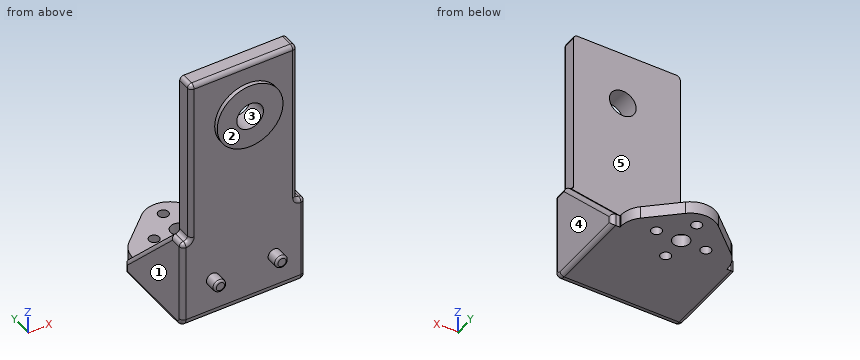
from build123d import *

# Parameters (mm, degrees)
SKETCH1_R           = 2
SKETCH1_R_2         = 1.25
BOSS_EXTRUDE1_DEPTH = 3
SKETCH2_W           = 26
SKETCH2_H           = 4
BOSS_EXTRUDE2_DEPTH = 60
SKETCH3_R           = 3.25
CUT_EXTRUDE1_DEPTH  = 72.226350639
SKETCH4_R           = 8
SKETCH4_R_2         = 3.25
BOSS_EXTRUDE3_DEPTH = 1
SKETCH5_R           = 1.5
BOSS_EXTRUDE4_DEPTH = 3
BOSS_EXTRUDE5_DEPTH = 2
FILLET1_R           = 2
FILLET2_R           = 1
FILLET3_R           = 0.5


# Some blends are built 0.0001 mm under size
with BuildPart() as part:
    # Sketch1 → Boss-Extrude1 (new body)
    with BuildSketch(Plane.XY):
        with BuildLine():
            Line((-13, -2.68256679), (-13, -25))
            Line((-13, -25), (13, -25))
            Line((13, -25), (13, -2.68256679))
            ThreePointArc((13, -2.68256679), (12.477468733, -0.233620837), (11.000887907, 1.788774838))
            Line((11.000887907, 1.788774838), (4.000887907, 8.052267471))
            ThreePointArc((4.000887907, 8.052267471), (0, 9.580925842), (-4.000887907, 8.052267471))
            Line((-4.000887907, 8.052267471), (-11.000887907, 1.788774838))
            ThreePointArc((-11.000887907, 1.788774838), (-12.477468733, -0.233620837), (-13, -2.68256679))
        make_face()
        Circle(SKETCH1_R, mode=Mode.SUBTRACT)
        with Locations((-6, 0)):
            Circle(SKETCH1_R_2, mode=Mode.SUBTRACT)
        with Locations((0, 6)):
            Circle(SKETCH1_R_2, mode=Mode.SUBTRACT)
        with Locations((6, 0)):
            Circle(SKETCH1_R_2, mode=Mode.SUBTRACT)
        with Locations((0, -6)):
            Circle(SKETCH1_R_2, mode=Mode.SUBTRACT)
    extrude(amount=BOSS_EXTRUDE1_DEPTH)

    # Sketch2 → Boss-Extrude2 (add)
    with BuildSketch(Plane.XY.offset(3)):
        with Locations((0, -23)):
            Rectangle(SKETCH2_W, SKETCH2_H)
    extrude(amount=BOSS_EXTRUDE2_DEPTH)

    # Sketch3 → Cut-Extrude1 (cut, through all)
    with BuildSketch(Plane(origin=(0, -21, 0), x_dir=(1, 0, 0), z_dir=(0, 1, 0))):
        with Locations(Location((1, -50, 0), (0, 0, 270))):
            Circle(SKETCH3_R)
    extrude(amount=-CUT_EXTRUDE1_DEPTH, mode=Mode.SUBTRACT)

    # Sketch4 → Boss-Extrude3 (add)
    with BuildSketch(Plane.XZ.offset(25)):
        with Locations(Location((1, 50, 0), (0, 0, 180))):
            Circle(SKETCH4_R)
        with Locations(Location((1, 50, 0), (0, 0, 90))):
            Circle(SKETCH4_R_2, mode=Mode.SUBTRACT)
    extrude(amount=BOSS_EXTRUDE3_DEPTH)

    # Sketch5 → Boss-Extrude4 (add)
    with BuildSketch(Plane.XZ.offset(25)):
        with Locations(Location((-7.5, 10, 0), (0, 0, 180))):
            Circle(SKETCH5_R)
        with Locations(Location((7.5, 10, 0), (0, 0, 180))):
            Circle(SKETCH5_R)
    extrude(amount=BOSS_EXTRUDE4_DEPTH)

    # Sketch6 → Boss-Extrude5 (add)
    with BuildSketch(Plane.ZY.offset(13)):
        Polygon((0, -3), (3, -3), (22, -21), (22, -25), (0, -25), align=None)
    boss_extrude5 = extrude(amount=BOSS_EXTRUDE5_DEPTH)

    # Mirror1: Boss-Extrude5 across plane
    add(boss_extrude5.mirror(Plane(origin=(0, 0, 0), x_dir=(0, 0, 1), z_dir=(1, 0, 0))))

    # Fillet1
    fillet1_edges = [part.edges().sort_by_distance(p)[0] for p in [
        (0, -25, 0),
        (0, -21, 3),
    ]]
    fillet(fillet1_edges, radius=FILLET1_R)

    # Fillet2
    # the kernel refuses this fillet: 1 mm, written as the material it adds along each edge
    with BuildSketch(Plane(origin=(13, -21, 22), x_dir=(1, 0, 0), z_dir=(0, -1, 0)), Plane(origin=(-13, -21, 22), x_dir=(0, 0, 1), z_dir=(0, -1, 0))) as fillet2_piece_1:
        with BuildLine():
            CenterArc((FILLET2_R, FILLET2_R), FILLET2_R, 180, 90)
            Line((0, FILLET2_R), (-FILLET2_R * 0.02, FILLET2_R))
            Line((-FILLET2_R * 0.02, FILLET2_R), (-FILLET2_R * 0.02, -FILLET2_R * 0.02))
            Line((-FILLET2_R * 0.02, -FILLET2_R * 0.02), (FILLET2_R, -FILLET2_R * 0.02))
            Line((FILLET2_R, -FILLET2_R * 0.02), (FILLET2_R, 0))
        make_face()
    extrude(amount=4)
    fillet2_2_edges = [part.edges().sort_by_distance(p)[0] for p in [
        (15, -13, 0),
        (15, -3, 1.5),
        (15, -12, 12.5),
        (15, -23, 22),
        (15, -25, 12),
        (-15, -25, 12),
        (15, -24.414213562, 0.585786438),
        (-15, -24.414213562, 0.585786438),
        (-13, -23, 63),
        (0, -25, 63),
        (13, -23, 63),
        (-15, -13, 0),
        (-15, -23, 22),
        (-15, -12, 12.5),
        (-15, -3, 1.5),
    ]]
    fillet(fillet2_2_edges, radius=FILLET2_R - 0.0001)  # a hair under: the kernel refuses the full size
    # the kernel refuses this fillet: 1 mm, written as the material it takes off along each edge
    with BuildSketch(Plane(origin=(-15, -24, 21), x_dir=(0, -1, 0), z_dir=(0, 0, -1))) as fillet2_3_piece_1:
        with BuildLine():
            CenterArc((0.0001, -0.9999), 0.9999, 0, 90)
            Line((1, -0.9999), (1, 0))
            Line((1, 0), (0.0001, 0))
        make_face()
    revolve(axis=Axis((-15, -24, 21), (-1, 0, 0)), revolution_arc=90, mode=Mode.SUBTRACT)
    with BuildSketch(Plane(origin=(12, -24, 63), x_dir=(0, -1, 0), z_dir=(-1, 0, 0))) as fillet2_3_piece_2:
        with BuildLine():
            CenterArc((0.0001, -0.9999), 0.9999, 0, 90)
            Line((1, -0.9999), (1, 0))
            Line((1, 0), (0.0001, 0))
        make_face()
    revolve(axis=Axis((12, -24, 63), (0, 0, 1)), revolution_arc=90, mode=Mode.SUBTRACT)
    with BuildSketch(Plane(origin=(-12, -24, 63), x_dir=(-1, 0, 0), z_dir=(0, 1, 0))) as fillet2_3_piece_3:
        with BuildLine():
            CenterArc((0.0001, -0.9999), 0.9999, 0, 90)
            Line((1, -0.9999), (1, 0))
            Line((1, 0), (0.0001, 0))
        make_face()
    revolve(axis=Axis((-12, -24, 63), (0, 0, 1)), revolution_arc=90, mode=Mode.SUBTRACT)
    with BuildSketch(Plane(origin=(15, -24, 21), x_dir=(0, 0, 1), z_dir=(0, 1, 0))) as fillet2_3_piece_4:
        with BuildLine():
            CenterArc((0.0001, -0.9999), 0.9999, 0, 90)
            Line((1, -0.9999), (1, 0))
            Line((1, 0), (0.0001, 0))
        make_face()
    revolve(axis=Axis((15, -24, 21), (1, 0, 0)), revolution_arc=90, mode=Mode.SUBTRACT)
    with BuildSketch(Plane(origin=(14, -25, 22), x_dir=(0, 0, -1), z_dir=(1, 0, 0))) as fillet2_3_piece_5:
        with BuildLine():
            CenterArc((FILLET2_R, FILLET2_R), FILLET2_R, 180, 90)
            Line((0, FILLET2_R), (-FILLET2_R * 0.02, FILLET2_R))
            Line((-FILLET2_R * 0.02, FILLET2_R), (-FILLET2_R * 0.02, -FILLET2_R * 0.02))
            Line((-FILLET2_R * 0.02, -FILLET2_R * 0.02), (FILLET2_R, -FILLET2_R * 0.02))
            Line((FILLET2_R, -FILLET2_R * 0.02), (FILLET2_R, 0))
        make_face()
    extrude(amount=1, mode=Mode.SUBTRACT)
    with BuildSketch(Plane(origin=(-13, -25, 23), x_dir=(1, 0, 0), z_dir=(0, 0, 1))) as fillet2_3_piece_6:
        with BuildLine():
            CenterArc((FILLET2_R, FILLET2_R), FILLET2_R, 180, 90)
            Line((0, FILLET2_R), (-FILLET2_R * 0.02, FILLET2_R))
            Line((-FILLET2_R * 0.02, FILLET2_R), (-FILLET2_R * 0.02, -FILLET2_R * 0.02))
            Line((-FILLET2_R * 0.02, -FILLET2_R * 0.02), (FILLET2_R, -FILLET2_R * 0.02))
            Line((FILLET2_R, -FILLET2_R * 0.02), (FILLET2_R, 0))
        make_face()
    extrude(amount=40, mode=Mode.SUBTRACT)
    with BuildSketch(Plane(origin=(13, -25, 23), x_dir=(-1, 0, 0), z_dir=(0, 0, 1))) as fillet2_3_piece_7:
        with BuildLine():
            CenterArc((FILLET2_R, -FILLET2_R), FILLET2_R, 90, 90)
            Line((0, -FILLET2_R), (-FILLET2_R * 0.02, -FILLET2_R))
            Line((-FILLET2_R * 0.02, -FILLET2_R), (-FILLET2_R * 0.02, FILLET2_R * 0.02))
            Line((-FILLET2_R * 0.02, FILLET2_R * 0.02), (FILLET2_R, FILLET2_R * 0.02))
            Line((FILLET2_R, FILLET2_R * 0.02), (FILLET2_R, 0))
        make_face()
    extrude(amount=40, mode=Mode.SUBTRACT)
    with BuildSketch(Plane(origin=(-14, -25, 22), x_dir=(0, 0, -1), z_dir=(-1, 0, 0))) as fillet2_3_piece_8:
        with BuildLine():
            CenterArc((FILLET2_R, -FILLET2_R), FILLET2_R, 90, 90)
            Line((0, -FILLET2_R), (-FILLET2_R * 0.02, -FILLET2_R))
            Line((-FILLET2_R * 0.02, -FILLET2_R), (-FILLET2_R * 0.02, FILLET2_R * 0.02))
            Line((-FILLET2_R * 0.02, FILLET2_R * 0.02), (FILLET2_R, FILLET2_R * 0.02))
            Line((FILLET2_R, FILLET2_R * 0.02), (FILLET2_R, 0))
        make_face()
    extrude(amount=1, mode=Mode.SUBTRACT)
    with BuildSketch(Plane(origin=(-14, -25, 23), x_dir=(1, 0, 0), z_dir=(0, 0, 1))) as fillet2_3_piece_9:
        with BuildLine():
            CenterArc((1 + FILLET2_R, FILLET2_R), FILLET2_R, 180, 90)
            Line((1 + FILLET2_R, 0), (1 + FILLET2_R, -FILLET2_R * 0.02))
            Line((1 + FILLET2_R, -FILLET2_R * 0.02), (1 - FILLET2_R * 0.02, -FILLET2_R * 0.02))
            Line((1 - FILLET2_R * 0.02, -FILLET2_R * 0.02), (1 - FILLET2_R * 0.02, FILLET2_R))
            Line((1 - FILLET2_R * 0.02, FILLET2_R), (1, FILLET2_R))
        make_face()
    revolve(axis=Axis((-14, -25, 23), (0, 1, 0)), revolution_arc=90, mode=Mode.SUBTRACT)
    with BuildSketch(Plane(origin=(14, -25, 23), x_dir=(0, 0, -1), z_dir=(1, 0, 0))) as fillet2_3_piece_10:
        with BuildLine():
            CenterArc((1 + FILLET2_R, FILLET2_R), FILLET2_R, 180, 90)
            Line((1 + FILLET2_R, 0), (1 + FILLET2_R, -FILLET2_R * 0.02))
            Line((1 + FILLET2_R, -FILLET2_R * 0.02), (1 - FILLET2_R * 0.02, -FILLET2_R * 0.02))
            Line((1 - FILLET2_R * 0.02, -FILLET2_R * 0.02), (1 - FILLET2_R * 0.02, FILLET2_R))
            Line((1 - FILLET2_R * 0.02, FILLET2_R), (1, FILLET2_R))
        make_face()
    revolve(axis=Axis((14, -25, 23), (0, 1, 0)), revolution_arc=90, mode=Mode.SUBTRACT)

    # Fillet3
    fillet3_edges = [part.edges().sort_by_distance(p)[0] for p in [
        (-6, -28, 10),
        (9, -28, 10),
    ]]
    fillet(fillet3_edges, radius=FILLET3_R)


solid = part.part
Can you work these out from the model? Positions are in its coordinate system, mm. Face numbers are marked on the shaded views. A direction names the side the tool comes from. Coordinates: 2 decimals unless noted, no trailing zeros. Order: outer loops, then holes, each group sorted by start corner. A loop starts at its lowest first (then second) coordinate and runs counter-clockwise, first axis right, second up. Notation, with made-up numbers: M -16.75,74 L 1.25,74 A16 ccw 1.25,102 Z; hole C 52.5,-3 d5. An arc over 180 degrees is marked long. Answer as CSV lines item,"result".
(1) On a 3-axis mill with a long thin cutter (end or side, diameter ignored), from which of +Z, -Z, +X, -X, +Y, -Y can I reach the whole of each face in a straight line? I mean the marked faces 4 and 5. Say none if no direction works.
Geometry check:
face 4,"+Z, -Z, +X, +Y, -Y"
face 5,"+Z, +Y"
(2) Suppose I cut it at C-C on z = 27.5. Please give me the cut outline in (x, y), plus the area to 3 significant figures.
Geometry check:
outline,"M -13,-24 A1 ccw -12,-25 L 12,-25 A1 ccw 13,-24 L 13,-21 L -13,-21 Z"
area,"104 mm^2"
(3) Suppose I cut it at B-B on y = 0. Please give me the cut outline in (x, z).
Geometry check:
outline,"M -12.37,0 L -7.25,0 L -7.25,3 L -12.37,3 Z; M -4.75,0 L -2,0 L -2,3 L -4.75,3 Z; M 2,0 L 4.75,0 L 4.75,3 L 2,3 Z; M 7.25,0 L 12.37,0 L 12.37,3 L 7.25,3 Z"
(4) If we mould it in two halves opening along X, with no side actions, what happens to the marked faces 1, 2 and 3? For each: released by +X, released by -X, zero draft, split by the parting line, or undercut.
Geometry check:
face 1,"released by -X"
face 2,"zero draft"
face 3,"undercut"
(5) I'm going to push flat-ended pins straight in: pin 1 (4 mm diameter, centred on x = 6, y = 0, fed in from +Z); pin 2 (3 mm diameter, centred on x = -7, z = 6.5, fed in from +Y); pin 3 (2 mm diameter, centred on y = -16.5, z = 18, fed in from -X). Where does each tip first touch, or does it pass through?
Geometry check:
pin 1,"z = 3"
pin 2,"y = -21"
pin 3,"x = -14.86"
(6) Please list where these lines run through material, in increasing order: L1, parallel to X at y = -11, z = 5; L2, parallel to Y at x = 0, z = 1.6; L3, parallel to Y at x = 0, z = 1.1.
Geometry check:
L1,"-15 to -13, 13 to 15"
L2,"-24.96 to -7.25, -4.75 to -2, 2 to 4.75, 7.25 to 9.58"
L3,"-24.79 to -7.25, -4.75 to -2, 2 to 4.75, 7.25 to 9.58"
(7) Suppose I cut it at A-A on x = 0. Count the separate pieces of the cut face and the enclosed holes in it, plus the area to 3 significant figures.
Geometry check:
separate pieces,"5"
enclosed holes,"0"
area,"301 mm^2"
